Here's how the part is built. I have some questions about the finished solid (model axes, mm). Face numbers are marked on the shaded views. A direction names the side the tool comes from. Round coordinates to 2 decimals unless told otherwise and drop trailing zeros. Loops run counter-clockwise (first coordinate to the right, second up) from the corner with the lowest first, then second, coordinate; pieces in that order, holes last. Notation, with made-up numbers: M 60.5,-28 L 98.5,-28 A36 ccw 98.5,11 Z; hole C 77.25,28 d11. An arc over 180 degrees is marked long. Use a Markdown table: item, result.
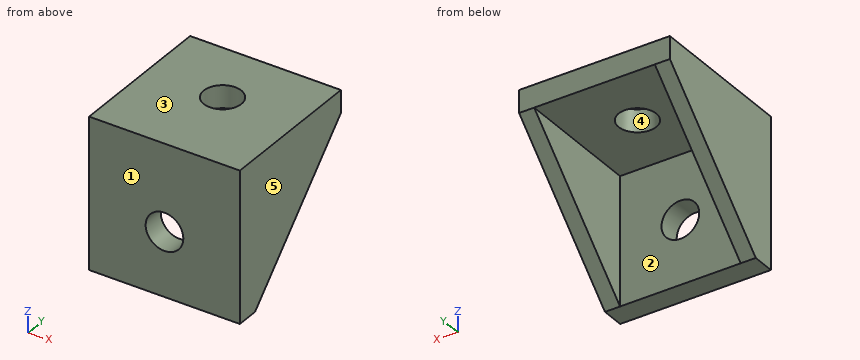
```python
from build123d import *

# Parameters (mm, degrees)
CROQUIS1_W                 = 20
CROQUIS1_H                 = 20
SALIENTE_EXTRUIR1_DEPTH    = 3
SALIENTE_EXTRUIR2_START    = 10
CROQUIS3_W                 = 20
CROQUIS3_H                 = 20
SALIENTE_EXTRUIR2_DEPTH    = 3
SALIENTE_EXTRUIR3_START    = 10
SALIENTE_EXTRUIR3_DEPTH    = 2
SALIENTE_EXTRUIR4_START    = -10
SALIENTE_EXTRUIR4_DEPTH    = 2
CROQUIS6_R                 = 2.5
CORTAR_EXTRUIR3_DEPTH      = 21
CORTAR_EXTRUIR3_DEPTH_BACK = 1
CROQUIS7_R                 = 2.5
CORTAR_EXTRUIR4_DEPTH      = 11
CORTAR_EXTRUIR4_DEPTH_BACK = 11


with BuildPart() as part:
    # Croquis1 → Saliente-Extruir1 (new body)
    with BuildSketch(Plane(origin=(0, 0, 0), x_dir=(1, 0, 0), z_dir=(0, 1, 0))):
        Rectangle(CROQUIS1_W, CROQUIS1_H)
    extrude(amount=SALIENTE_EXTRUIR1_DEPTH)

    # Croquis3 → Saliente-Extruir2 (add)
    with BuildSketch(Plane.XY.offset(SALIENTE_EXTRUIR2_START)):
        with Locations((0, 10)):
            Rectangle(CROQUIS3_W, CROQUIS3_H)
    extrude(amount=-SALIENTE_EXTRUIR2_DEPTH)

    # Croquis4 → Saliente-Extruir3 (add)
    with BuildSketch(Plane(origin=(0, 0, 0), x_dir=(0, 0, -1), z_dir=(1, 0, 0)).offset(SALIENTE_EXTRUIR3_START)):
        Polygon((-7, 20), (10, 3), (-7, 3), align=None)
    extrude(amount=-SALIENTE_EXTRUIR3_DEPTH)

    # Croquis8 → Saliente-Extruir4 (add)
    with BuildSketch(Plane(origin=(0, 0, 0), x_dir=(0, 0, -1), z_dir=(1, 0, 0)).offset(SALIENTE_EXTRUIR4_START)):
        Polygon((10, 3), (-7, 20), (-7, 3), align=None)
    extrude(amount=SALIENTE_EXTRUIR4_DEPTH)

    # Croquis6 → Cortar-Extruir3 (cut, two sides)
    with BuildSketch(Plane(origin=(0, 0, 0), x_dir=(1, 0, 0), z_dir=(0, 1, 0))) as cortar_extruir3_sk:
        with Locations((0, 1.5)):
            Circle(CROQUIS6_R)
    extrude(amount=CORTAR_EXTRUIR3_DEPTH, mode=Mode.SUBTRACT)
    extrude(cortar_extruir3_sk.sketch, amount=-CORTAR_EXTRUIR3_DEPTH_BACK, mode=Mode.SUBTRACT)

    # Croquis7 → Cortar-Extruir4 (cut, two sides)
    with BuildSketch(Plane.XY) as cortar_extruir4_sk:
        with Locations((0, 11.5)):
            Circle(CROQUIS7_R)
    extrude(amount=CORTAR_EXTRUIR4_DEPTH, mode=Mode.SUBTRACT)
    extrude(cortar_extruir4_sk.sketch, amount=-CORTAR_EXTRUIR4_DEPTH_BACK, mode=Mode.SUBTRACT)


solid = part.part
```
Q1. Will these pins go through, and if not, where does the flat tip stop? P1, Ø1.5, axis at x = 5.5, y = 11, coming from the -Z side; P2, Ø10, axis at x = 4.5, y = 10, coming from the -Z side; P3, Ø1, axis at x = -0.5, z = 3, coming from the +Y side.
Return value:
| item | result |
|---|---|
| P1 | stops at z = 7 |
| P2 | stops at z = -6.57 |
| P3 | stops at y = 3 |
Q2. For the marked faces 1 and 2, which set-ups out of +Z, -Z, +X, -X, +Y, -Y let a thin tool reach every point of the face, with its end or its side?
Return value:
| item | result |
|---|---|
| face 1 | +Z, -Z, +X, -X, -Y |
| face 2 | -Z, +Y |
Q3. Imagine slicing it at D-D, the plane x = 5.5. Please give me the cut outline in (y, z), then the cut area to 3 significant figures.
Return value:
| item | result |
|---|---|
| outline | M 0,-10 L 3,-10 L 3,7 L 20,7 L 20,10 L 0,10 Z |
| area | 111 mm^2 |
Q4. We'd pull the mould along X, two halves only. Please class the marked faces 3, 4 and 5: pulls with the +X half, pulls with the -X half, needs draft (parallel to the pull), parting line crosses it, or undercut.
Return value:
| item | result |
|---|---|
| face 3 | needs draft |
| face 4 | undercut |
| face 5 | pulls with the +X half |
Q5. Imagine slicing it at C-C, the plane y = 18.75. Please give me the cut outline in (x, z), then the cut area to 3 significant figures.
Return value:
| item | result |
|---|---|
| outline | M -10,5.75 L -8,5.75 L -8,7 L 8,7 L 8,5.75 L 10,5.75 L 10,10 L -10,10 Z |
| area | 65.0 mm^2 |
Q6. Imagine slicing it at B-B, the plane x = -1.5. Please give me the cut outline in (y, z).
Return value:
| item | result |
|---|---|
| outline | M 0,-10 L 3,-10 L 3,-3.5 L 0,-3.5 Z; M 0,0.5 L 3,0.5 L 3,7 L 9.5,7 L 9.5,10 L 0,10 Z; M 13.5,7 L 20,7 L 20,10 L 13.5,10 Z |
Q7. Imagine slicing it at A-A, the plane z = -1.5. Please give me the cut outline in (x, y).
Return value:
| item | result |
|---|---|
| outline | M -10,0 L -2.5,0 L -2.5,3 L -8,3 L -8,11.5 L -10,11.5 Z; M 2.5,0 L 10,0 L 10,11.5 L 8,11.5 L 8,3 L 2.5,3 Z |
Q8. I need wall thicknesses on line 1 (X direction, y = 11.5, z = 7.95); line 2 (X direction, y = 5.5, z = -6.25); line 3 (Y direction, x = 0, z = 8.05). Which ranges of each line are inside material? Lowest first, please. Write a range as from..to.
Return value:
| item | result |
|---|---|
| line 1 | x = -10..-2.5, 2.5..10 |
| line 2 | x = -10..-8, 8..10 |
| line 3 | y = 0..9, 14..20 |
